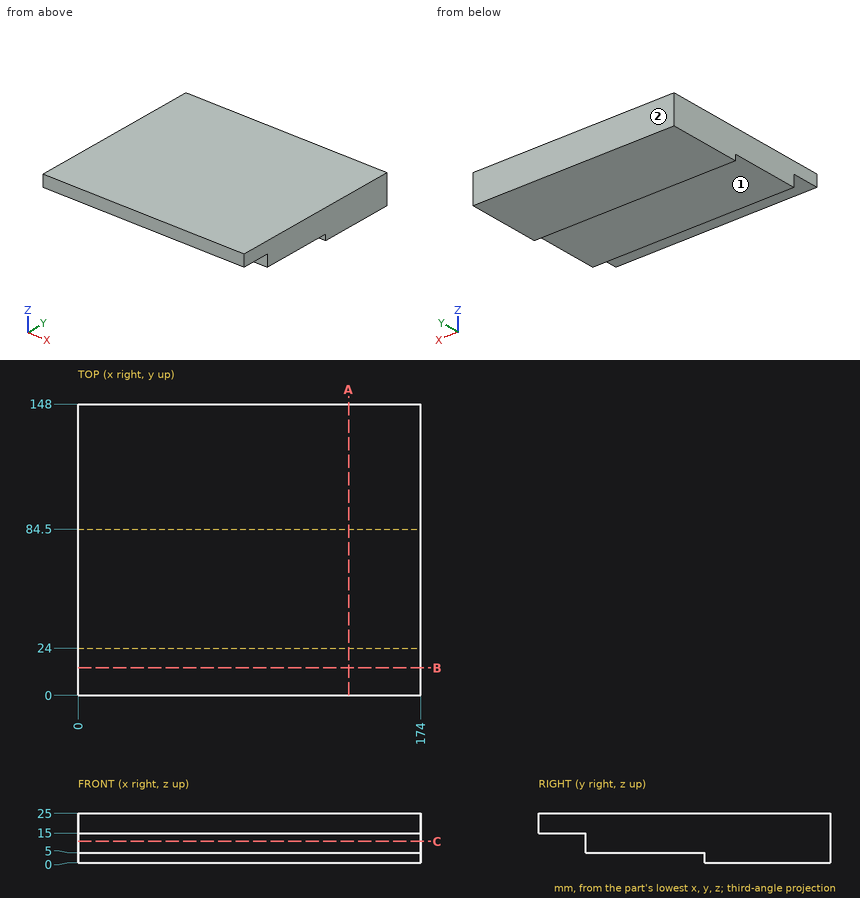
Check sheet for the drawn part. Datum: minimum x, y, z corner. Units: mm. A direction names the side the tool comes from. Round coordinates to 2 decimals unless told otherwise and drop trailing zeros. Loops run counter-clockwise (first coordinate to the right, second up) from the corner with the lowest first, then second, coordinate; pieces in that order, holes last. Notation, with made-up numbers: (60.5, 85) - (98.5, 85) arc R25 ccw to (98.5, 118) - close; hole circle Ø11 at (49.25, -27.75). An arc over 180 degrees is marked (long way). Write item = value, one per line. Start each with the question number.
1. Section check C-C on z = 10.75. Enter the section's corners in (x, y), then the cut area to 3 significant figures.
2. Section check A-A on x = 137.5. Enter the section's corners in (y, z), then the cut area to 3 significant figures.
3. Section check B-B on y = 14. Enter the section's corners in (x, z), then the cut area to 3 significant figures.
4. Depth check by flat-ended pin: pin 1 (5 mm diameter, centred on x = 107.5, z = 20.5, fed in from -Y); pin 2 (4 mm diameter, centred on x = 121, z = 2.5, fed in from -Y); pin 3 (19 mm diameter, centred on x = 116, y = 16.5, fed in from -Z); pin 4 (3 mm diameter, centred on x = 111.5, z = 11, fed in from -Y). Enter the tip coordinate at first touch or a pass-through.
5. Thickness scan on line 1 (Z direction, x = 10, y = 38); line 2 (Z direction, x = 74, y = 22.5); line 3 (Y direction, x = 98.5, z = 3.25). Record the ranges inside material, lowest first.
6. Set-up check for the marked faces 1 and 2: record each of +Z, -Z, +X, -X, +Y, -Y from which the full face is reachable in a straight line by a thin tool's end or side.
Working result:
q1.outline = (0, 24) - (174, 24) - (174, 148) - (0, 148) - close
q1.area = 21,600 mm^2
q2.outline = (0, 15) - (24, 15) - (24, 5) - (84.5, 5) - (84.5, 0) - (148, 0) - (148, 25) - (0, 25) - close
q2.area = 3,040 mm^2
q3.outline = (0, 15) - (174, 15) - (174, 25) - (0, 25) - close
q3.area = 1,740 mm^2
q4.pin_1 = 0
q4.pin_2 = 84.5
q4.pin_3 = 5
q4.pin_4 = 24
q5.line_1 = 5 to 25
q5.line_2 = 15 to 25
q5.line_3 = 84.5 to 148
q6.face_1 = -Z, +X, -X, -Y
q6.face_2 = +Z, -Z, +X, -X, +Y
